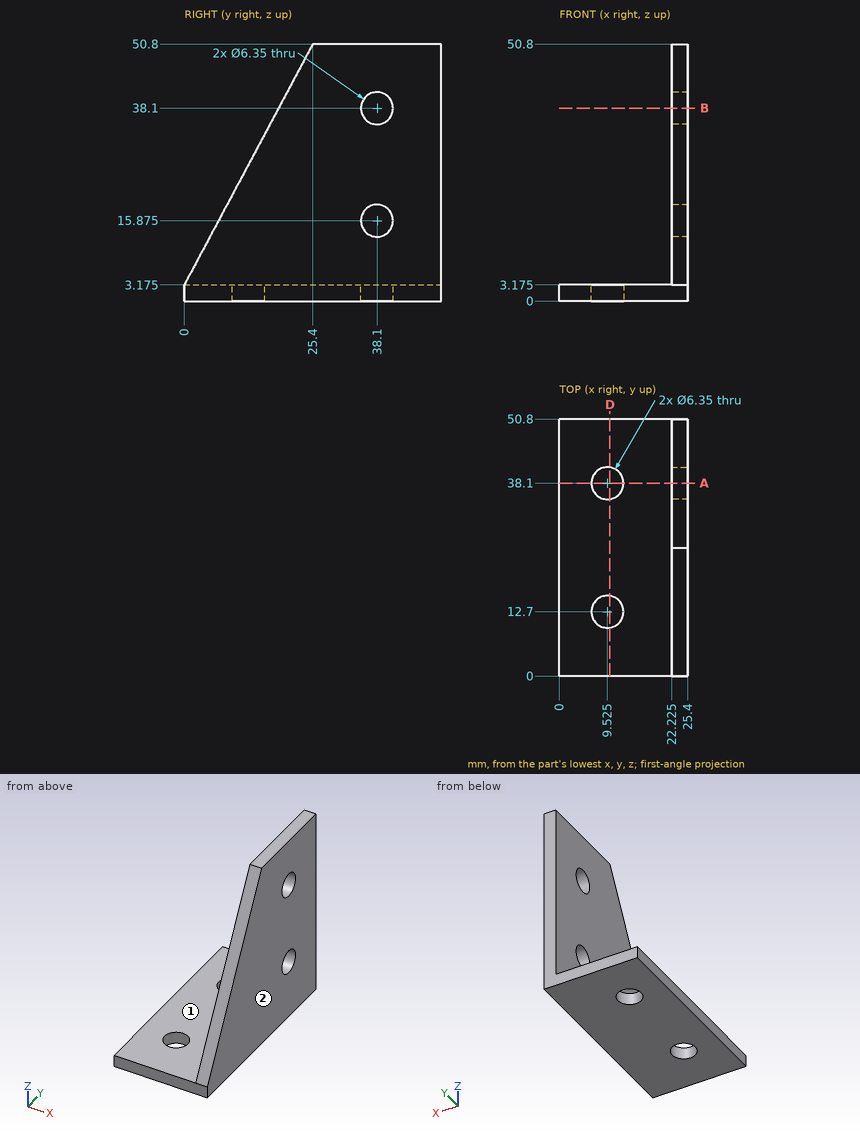
Study the drawing (mm; zero at the part's minimum x, y, z) and answer. A direction names the side the tool comes from. Give positions to 0.01 mm unless a question says otherwise; leave off trailing zeros. Loops run counter-clockwise (first coordinate to the right, second up) from the corner with the lowest first, then second, coordinate; pieces in that order, holes last. Notation, with made-up numbers: M -6,-23.5 L 40,-23.5 A23 ccw 40,-2.5 Z; hole C 53.5,30 d5. An arc over 180 degrees is marked long. Use CSV: the item, a comma, the result in double quotes.
1) Given P1, Ø12, axis at x = 14.5, z = 32.5, coming from the +Y side; P2, Ø5, axis at x = 13, y = 23, coming from the +Z side (3 decimals); P3, Ø3, axis at y = 10.5, z = 7.5, coming from the -X side (3 decimals), each flat-ended and moving along its own axis, determine where each tip first touches the part or whether it passes through.
Answer:
P1,"through"
P2,"z = 3.175"
P3,"x = 22.225"
2) Which of the six approach directions +Z, -Z, +X, -X, +Y, -Y give full straight-line access (tool end or side, diameter ignored) to the marked faces 1 and 2?
Answer:
face 1,"+Z, -X, +Y, -Y"
face 2,"+Z, -Z, +X, +Y, -Y"
3) Find section A-A on y = 38.1. Write down the section's boundary in (x, z) (3 decimals), plus the area to 3 significant figures.
Answer:
outline,"M 0,0 L 6.35,0 L 6.35,3.175 L 0,3.175 Z; M 12.7,0 L 25.4,0 L 25.4,12.7 L 22.225,12.7 L 22.225,3.175 L 12.7,3.175 Z; M 22.225,19.05 L 25.4,19.05 L 25.4,34.925 L 22.225,34.925 Z; M 22.225,41.275 L 25.4,41.275 L 25.4,50.8 L 22.225,50.8 Z"
area,"171 mm^2"
4) Find section B-B on z = 38.1. Write down the section's boundary in (x, y) (3 decimals), plus the area to 3 significant figures.
Answer:
outline,"M 22.225,18.627 L 25.4,18.627 L 25.4,34.925 L 22.225,34.925 Z; M 22.225,41.275 L 25.4,41.275 L 25.4,50.8 L 22.225,50.8 Z"
area,"82.0 mm^2"
5) Consider L1, parallel to Z at x = 24.4, y = 38.1 (3 decimals); L2, parallel to Z at x = 18.5, y = 31 (3 decimals); L3, parallel to X at y = 47.5, z = 43.5 (3 decimals). Determine where each line is inside the solid, lowest interval first.
Answer:
L1,"0 to 12.7, 19.05 to 34.925, 41.275 to 50.8"
L2,"0 to 3.175"
L3,"22.225 to 25.4"
6) Find section D-D on x = 10. Write down the section's boundary in (y, z) (3 decimals).
Answer:
outline,"M 0,0 L 9.561,0 L 9.561,3.175 L 0,3.175 Z; M 15.839,0 L 34.961,0 L 34.961,3.175 L 15.839,3.175 Z; M 41.239,0 L 50.8,0 L 50.8,3.175 L 41.239,3.175 Z"
